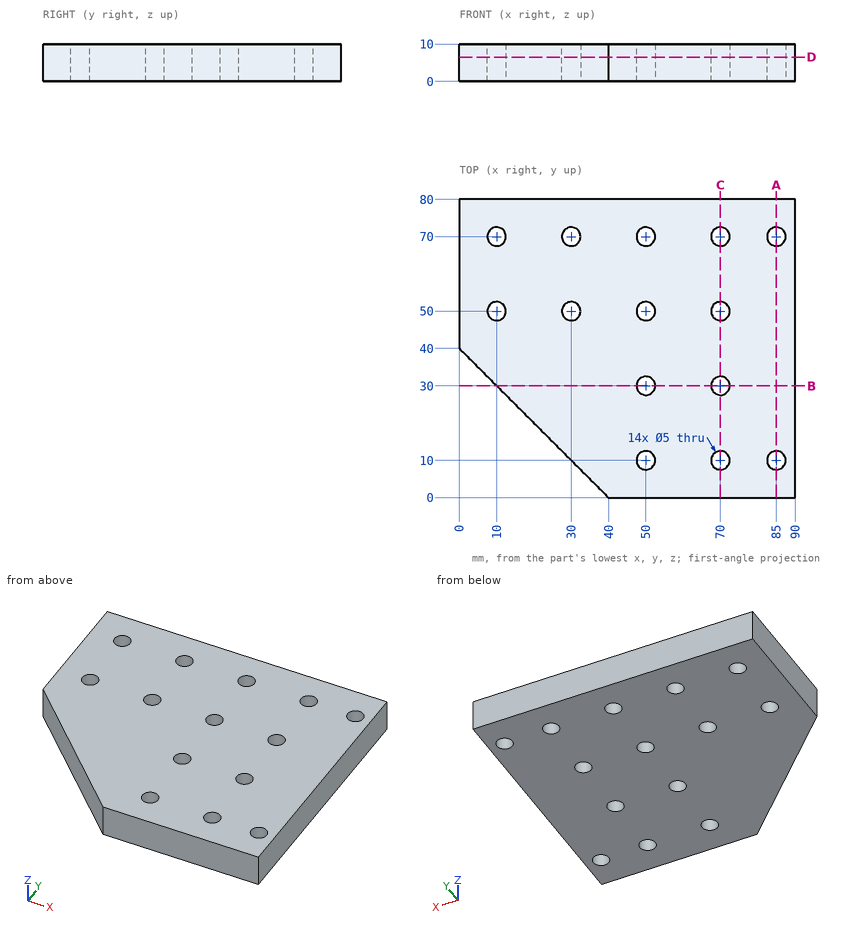
Source: three-view drawing plus pictorial views. Frame: mm from the lowest corner of the part. Round coordinates to 2 decimals unless told otherwise and drop trailing zeros. Loops run counter-clockwise (first coordinate to the right, second up) from the corner with the lowest first, then second, coordinate; pieces in that order, holes last. Notation, with made-up numbers: (73, 23.25) - (113, 23.25) arc R28 ccw to (113, 58.25) - close; hole circle Ø1 at (-39.5, -7.75). An arc over 180 degrees is marked (long way). Write item = value, one per line. Start each with the question number.
Item 1: First-contact query: pin 1 Ø4.5 at (x, y) = (70, 50) entering from -Z. Flat tip, straight axial feed; report the tip coordinate or a pass-through.
Item 2: Section query D-D on z = 6.5. Count the separate pieces of the cut face and the enclosed holes in it, plus the area to 3 significant figures.
Item 3: Material intervals for line 1 (Y direction, x = 50, z = 8); line 2 (Y direction, x = 30, z = 5.25); line 3 (Y direction, x = 28, z = 1.5), sorted ascending.
Item 4: Section query A-A on x = 85. Output: boundary loops of the cut face in (y, z), plus the area to 3 significant figures.
Item 5: Section query B-B on y = 30. Output: boundary loops of the cut face in (x, z), plus the area to 3 significant figures.
Item 6: Section query C-C on x = 70. Output: boundary loops of the cut face in (y, z), plus the area to 3 significant figures.
Results list:
q1.pin_1 = through
q2.separate_pieces = 1
q2.enclosed_holes = 14
q2.area = 6,130 mm²
q3.line_1 = 0 to 7.5, 12.5 to 27.5, 32.5 to 47.5, 52.5 to 67.5, 72.5 to 80
q3.line_2 = 10 to 47.5, 52.5 to 67.5, 72.5 to 80
q3.line_3 = 12 to 48.5, 51.5 to 68.5, 71.5 to 80
q4.outline = (0, 0) - (7.5, 0) - (7.5, 10) - (0, 10) - close; (12.5, 0) - (67.5, 0) - (67.5, 10) - (12.5, 10) - close; (72.5, 0) - (80, 0) - (80, 10) - (72.5, 10) - close
q4.area = 700 mm²
q5.outline = (10, 0) - (47.5, 0) - (47.5, 10) - (10, 10) - close; (52.5, 0) - (67.5, 0) - (67.5, 10) - (52.5, 10) - close; (72.5, 0) - (90, 0) - (90, 10) - (72.5, 10) - close
q5.area = 700 mm²
q6.outline = (0, 0) - (7.5, 0) - (7.5, 10) - (0, 10) - close; (12.5, 0) - (27.5, 0) - (27.5, 10) - (12.5, 10) - close; (32.5, 0) - (47.5, 0) - (47.5, 10) - (32.5, 10) - close; (52.5, 0) - (67.5, 0) - (67.5, 10) - (52.5, 10) - close; (72.5, 0) - (80, 0) - (80, 10) - (72.5, 10) - close
q6.area = 600 mm²
